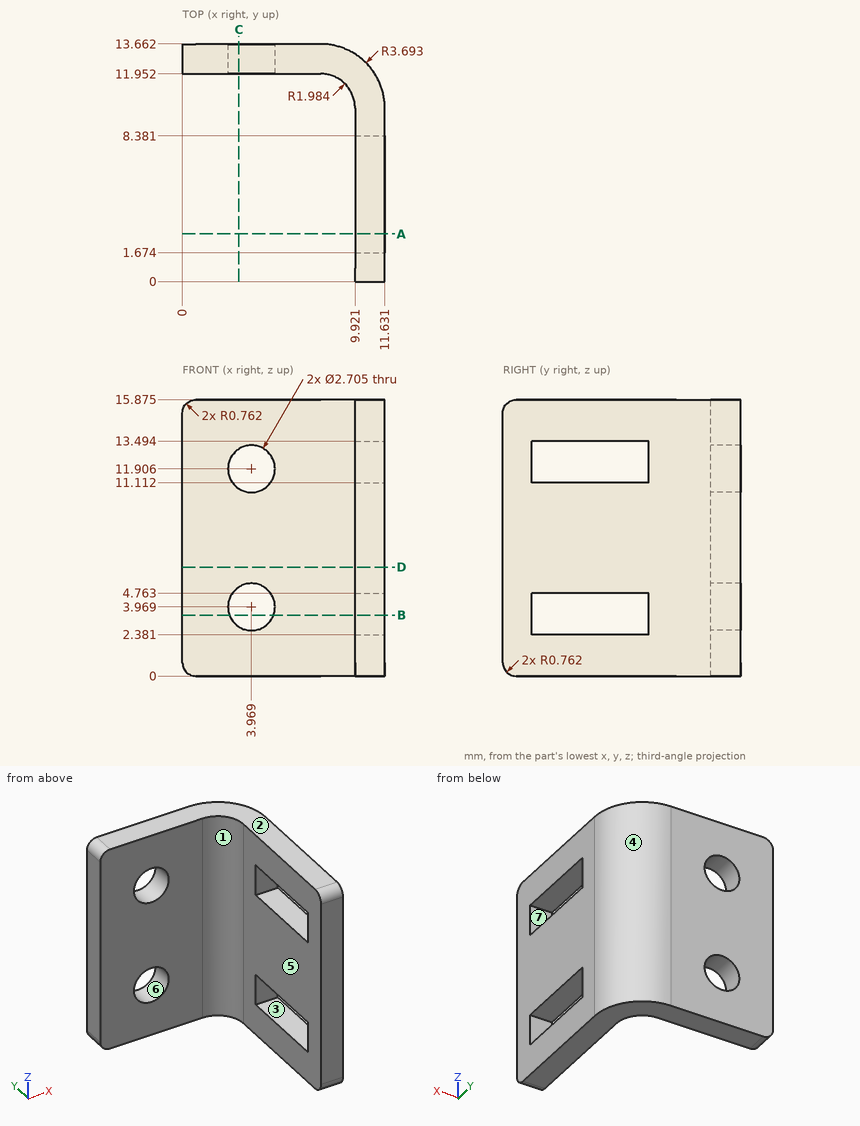
Check sheet for the drawn part. Datum: minimum x, y, z corner. Units: mm. A direction names the side the tool comes from. Coordinates: 2 decimals unless noted, no trailing zeros. Loops run counter-clockwise (first coordinate to the right, second up) from the corner with the lowest first, then second, coordinate; pieces in that order, holes last. Notation, with made-up numbers: (26.5, 24) - (40.5, 24) arc R20 cw to (40.5, 36) - close; hole circle Ø8 at (26, 28). An arc over 180 degrees is marked (long way). Put each result on its own line as item: value.
Item 1: Section check B-B (z = 3.5). Enter the section's corners in (x, y).
Conclusion:
outline: (0, 11.95) - (2.7, 11.95) - (2.7, 13.66) - (0, 13.66) - close; (5.24, 11.95) - (7.94, 11.95) arc R1.98 cw to (9.92, 9.97) - (9.92, 8.38) - (11.63, 8.38) - (11.63, 9.97) arc R3.69 ccw to (7.94, 13.66) - (5.24, 13.66) - close; (9.92, 0) - (11.63, 0) - (11.63, 1.67) - (9.92, 1.67) - close
Item 2: Section check C-C (x = 3.25). Enter the section's corners in (y, z) (1 decimal), then the cut area to 3 significant figures.
Conclusion:
outline: (12, 0) - (13.7, 0) - (13.7, 2.8) - (12, 2.8) - close; (12, 5.1) - (13.7, 5.1) - (13.7, 10.8) - (12, 10.8) - close; (12, 13.1) - (13.7, 13.1) - (13.7, 15.9) - (12, 15.9) - close
area: 19.3 mm2
Item 3: Draft check along Y on the marked faces 1, 2, 3 and 4. Enter one of: pulls with the +Y half, pulls with the -Y half, needs draft (parallel to the pull), parting line crosses it, or undercut.
Conclusion:
face 1: pulls with the -Y half
face 2: needs draft
face 3: undercut
face 4: pulls with the +Y half
Item 4: Section check A-A (y = 2.75). Enter the section's corners in (x, z) (1 decimal).
Conclusion:
outline: (9.9, 0) - (11.6, 0) - (11.6, 2.4) - (9.9, 2.4) - close; (9.9, 4.8) - (11.6, 4.8) - (11.6, 11.1) - (9.9, 11.1) - close; (9.9, 13.5) - (11.6, 13.5) - (11.6, 15.9) - (9.9, 15.9) - close
Item 5: Gauge pin test, flat ends, axial feed: pin 1 Ø1 at (x, z) = (8, 12.5) entering from -Y; pin 2 Ø1 at (x, z) = (2.5, 3) entering from -Y; pin 3 Ø5 at (x, z) = (7, 5) entering from -Y; pin 4 Ø3 at (x, y) = (8, 8) entering from -Z. Record the tip position at first contact, or that the pin passes through.
Conclusion:
pin 1: stops at y = 11.87
pin 2: stops at y = 11.95
pin 3: stops at y = 11.19
pin 4: passes through
Item 6: Set-up check for the marked faces 5, 6 and 7: record each of +Z, -Z, +X, -X, +Y, -Y from which the full face is reachable in a straight line by a thin tool's end or side.
Conclusion:
face 5: +Z, -Z, -X, -Y
face 6: +Y, -Y
face 7: +X, -X
Item 7: Scan lines: line 1 along Z through (x, y) = (10, 2.25) (1 decimal); line 2 along X through (y, z) = (9.75, 2); line 3 along Y through (x, z) = (4.5, 13.75). Record each from-to range of solid material in increasing order.
Conclusion:
line 1: z = 0 to 2.4, 4.8 to 11.1, 13.5 to 15.9
line 2: x = 9.92 to 11.63
line 3: y = 11.95 to 13.66
Item 8: Section check D-D (z = 6.25). Enter the section's corners in (x, y).
Conclusion:
outline: (0, 11.95) - (7.94, 11.95) arc R1.98 cw to (9.92, 9.97) - (9.92, 0) - (11.63, 0) - (11.63, 9.97) arc R3.69 ccw to (7.94, 13.66) - (0, 13.66) - close
